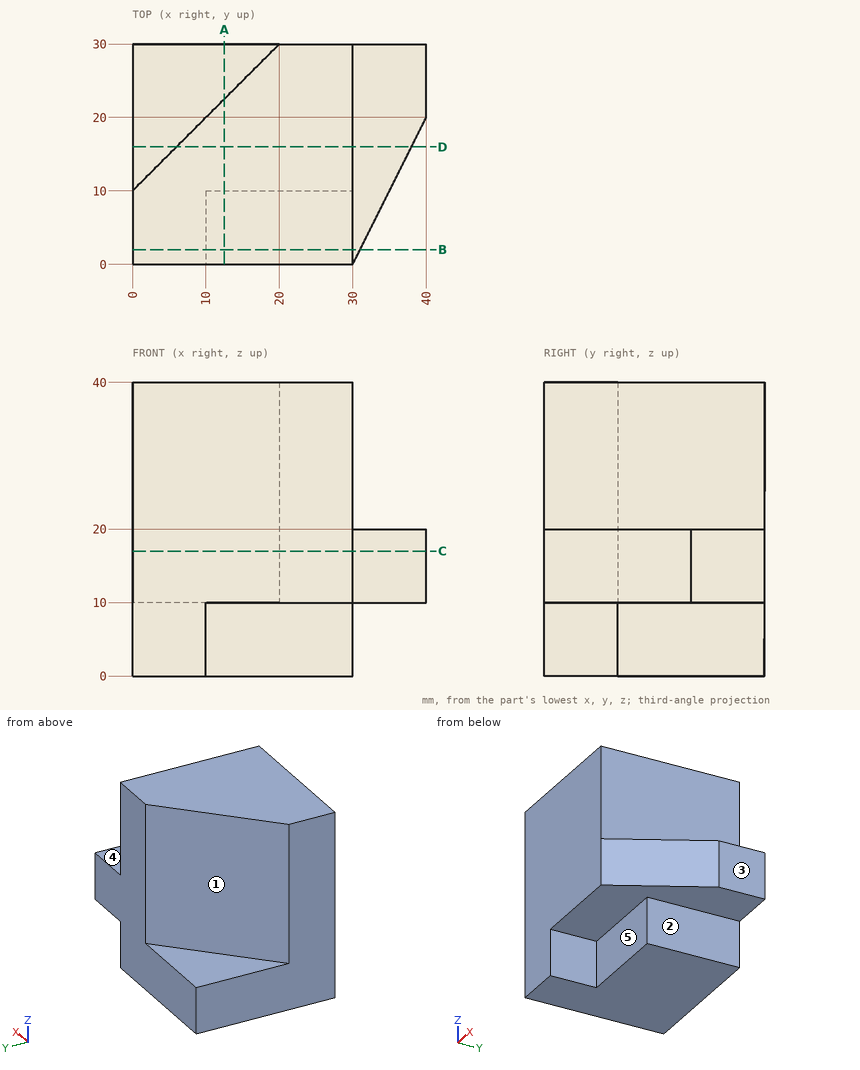
Here's the drawing with two shaded views (mm, measured from the low corner). I have some questions. A direction names the side the tool comes from. Coordinates: 2 decimals unless noted, no trailing zeros. Loops run counter-clockwise (first coordinate to the right, second up) from the corner with the lowest first, then second, coordinate; pieces in that order, holes last. Notation, with made-up numbers: M 75,22 L 118,22 A14 ccw 118,28 Z; hole C 77.25,-5 d5. An arc over 180 degrees is marked long. Answer as CSV lines item,"result". Start each with the question number.
1. If I drill on probe 1 along X at (y, z) = (6.5, 6); probe 2 along Z at (x, y) = (11, 9.5), over which ranges is the centre line in solid material (lowest first)? Write a range as [from, to].
2. Suppose I cut it at A-A, the plane x = 12.5. List the corners of the cut face in (y, z) for me.
3. Suppose I cut it at D-D, the plane y = 16. List the corners of the cut face in (x, z) for me.
4. Suppose I cut it at B-B, the plane y = 2. List the corners of the cut face in (x, z) for me.
5. Suppose I cut it at C-C, the plane z = 17. List the corners of the cut face in (x, y) for me, plus the area to 3 significant figures.
6. For pin 1 Ø1 at (y, z) = (14.5, 11.5) entering from -X; pin 2 Ø10 at (y, z) = (23.5, 32) entering from -X; pin 3 Ø3 at (x, z) = (14, 35.5) entering from +Y, each with a flat end and sliding along its axis, tell me the tip position at first contact or that it passes through.
7. For the marked faces 1, 2, 3, 4 and 5, which set-ups out of +Z, -Z, +X, -X, +Y, -Y let a thin tool reach every point of the face, with its end or its side?
Output:
1,probe 1,"x = [0, 10]"
1,probe 2,"z = [10, 40]"
2,outline,"M 0,10 L 10,10 L 10,0 L 30,0 L 30,10 L 22.5,10 L 22.5,40 L 0,40 Z"
3,outline,"M 0,0 L 30,0 L 30,10 L 38,10 L 38,20 L 30,20 L 30,40 L 6,40 L 6,10 L 0,10 Z"
4,outline,"M 0,0 L 10,0 L 10,10 L 31,10 L 31,20 L 30,20 L 30,40 L 0,40 Z"
5,outline,"M 0,0 L 30,0 L 40,20 L 40,30 L 20,30 L 0,10 Z"
5,area,"900 mm^2"
6,pin 1,"stops at x = 4"
6,pin 2,"stops at x = 8.5"
6,pin 3,"stops at y = 25.5"
7,face 1,"+Z, -X, +Y"
7,face 2,"-Z, +X, +Y, -Y"
7,face 3,"+Z, -Z, +X, +Y, -Y"
7,face 4,"+Z, +X, +Y, -Y"
7,face 5,"-Z, +X, -Y"
